```python
from build123d import *

# Parameters (mm, degrees)
PAD_DEPTH       = 9
POCKET_DEPTH    = 6
SKETCH002_W     = 26.5
SKETCH002_H     = 35
POCKET001_DEPTH = 6


with BuildPart() as part:
    # Sketch → Pad (new body)
    with BuildSketch(Plane.XY):
        with BuildLine():
            ThreePointArc((-65, 41), (-106, 0), (-65, -41))
            Line((-65, -41), (65, -41))
            ThreePointArc((65, -41), (106, 0), (65, 41))
            Line((-65, 41), (65, 41))
        make_face()
    extrude(amount=PAD_DEPTH)

    # Sketch001 (on Face6 of Pad) → Pocket (cut)
    with BuildSketch(Plane.XY.offset(9)):
        with BuildLine():
            ThreePointArc((-62.5, 6), (-68.5, 0), (-62.5, -6))
            Line((-62.5, -6), (62.5, -6))
            ThreePointArc((62.5, -6), (68.5, 0), (62.5, 6))
            Line((-62.5, 6), (62.5, 6))
        make_face()
    extrude(amount=-POCKET_DEPTH, mode=Mode.SUBTRACT)

    # Sketch002 (on Face5 of Pocket) → Pocket001 (cut)
    with BuildSketch(Plane.XY.offset(9)):
        with Locations((0, -23.5)):
            Rectangle(SKETCH002_W, SKETCH002_H)
    extrude(amount=-POCKET001_DEPTH, mode=Mode.SUBTRACT)


solid = part.part
```
For this review, take the finished solid that the model builds, in its own axes (mm). A direction names the side the tool comes from. Round coordinates to 2 decimals unless told otherwise and drop trailing zeros. Loops run counter-clockwise (first coordinate to the right, second up) from the corner with the lowest first, then second, coordinate; pieces in that order, holes last.
Q1. Machinability: for faces 5 (the face through (-13.25, -24, 6)), 6 (the face through (-1, 10, 9)), 7 (the face through (38, -6, 6)), which of the approach directions +Z, -Z, +X, -X, +Y, -Y give a long, thin tool a straight path to every point of the face, cutting with its end or side? Answer none if there is none.
Result sheet:
face 5: +Z, -Y
face 6: +Z, +X, -X, +Y, -Y
face 7: +Z
Q2. Add section B-B on y = 0. Write out the cut boundary in (x, z).
Result sheet:
outline: (-106, 0) - (106, 0) - (106, 9) - (68.5, 9) - (68.5, 3) - (-68.5, 3) - (-68.5, 9) - (-106, 9) - close
Q3. Add section D-D on y = 33.5. Write out the cut boundary in (x, z).
Result sheet:
outline: (-88.64, 0) - (88.64, 0) - (88.64, 9) - (-88.64, 9) - close
Q4. To check wall thickness, follow line 1 along Y through (x, z) = (46, 7.25); line 2 along Z through (x, y) = (-5, -7); line 3 along X through (y, z) = (-19.5, 8.5). State the ranges of each line that lie inside material, in increasing order.
Result sheet:
line 1: y = -41 to -6, 6 to 41
line 2: z = 0 to 3
line 3: x = -101.07 to -13.25, 13.25 to 101.07
Q5. Add section C-C on x = 8. Write out the cut boundary in (y, z).
Result sheet:
outline: (-41, 0) - (41, 0) - (41, 9) - (6, 9) - (6, 3) - (-41, 3) - close
Q6. Mouldability with a two-part tool opening along X and no side actions: class faces 1 (the face through (-1, 1, 0)), 2 (the face through (-105.99, 0.9, 4.44)), 3 (the face through (-68.5, 0.1, 6)), 4 (the face through (105.99, -0.9, 4.44)) as +X half, -X half, draft (parallel to the pull), parting line (faces both ways), or undercut.
Result sheet:
face 1: draft
face 2: -X half
face 3: undercut
face 4: +X half
Q7. Insertion check: pin 1 Ø5 at (y, z) = (-29, 6.5) entering from -X (3 decimals); pin 2 Ø5 at (y, z) = (-19.5, 4) entering from -X; pin 3 Ø3 at (y, z) = (-28, 5.5) entering from +X (3 decimals). Each pin has a flat end and moves straight along its axis. Give the tip position at first contact, or say it passes through.
Result sheet:
pin 1: stops at x = -96.285
pin 2: stops at x = -102.31
pin 3: stops at x = 96.285
Q8. Add section A-A on x = -41. Write out the cut boundary in (y, z).
Result sheet:
outline: (-41, 0) - (41, 0) - (41, 9) - (6, 9) - (6, 3) - (-6, 3) - (-6, 9) - (-41, 9) - close
